from build123d import *

# Parameters (mm, degrees)
SKETCH038_W        = 140
SKETCH038_H        = 93.9
PAD004_DEPTH       = 3
SKETCH039_W        = 12.5
SKETCH039_H        = 38.6472
POCKET028_DEPTH    = 3
SKETCH040_W        = 24
SKETCH040_H        = 60
POCKET029_DEPTH    = 1.5
SKETCH041_R        = 1.05
POCKET030_DEPTH    = 3.001
SKETCH042_R        = 1.9
POCKET031_DEPTH    = 1.4
CHAMFER001_1_ANGLE = 45
CHAMFER001_1_SIZE  = 0.843
CHAMFER001_2_ANGLE = 45
CHAMFER001_2_SIZE  = 0.843
CHAMFER001_3_ANGLE = 45
CHAMFER001_3_SIZE  = 0.843
CHAMFER001_4_ANGLE = 45
CHAMFER001_4_SIZE  = 0.843
FILLET004_R        = 1.5
SKETCH043_R        = 4.85
POCKET032_DEPTH    = 10
FILLET005_R        = 1.8
POCKET033_DEPTH    = 12


with BuildPart() as part:
    # Sketch038 (on XY_Plane154 of Origin468) → Pad004 (new body)
    with BuildSketch(Plane.XY):
        Rectangle(SKETCH038_W, SKETCH038_H)
    extrude(amount=PAD004_DEPTH)

    # Sketch039 (on Face6 of Pad004) → Pocket028 (cut)
    with BuildSketch(Plane.XY.offset(3)):
        Polygon((-61.3, 38.25), (-61.3, -19.25), (-4.3, -19.25), (-4.3, -38.25), (34.2, -38.25), (34.2, 38.25), align=None)
        with Locations((47.48708, -1.86296)):
            Rectangle(SKETCH039_W, SKETCH039_H)
    extrude(amount=-POCKET028_DEPTH, mode=Mode.SUBTRACT)

    # Sketch040 (on Face4 of Pocket028) → Pocket029 (cut)
    with BuildSketch(Plane(origin=(0, 0, 0), x_dir=(1, 0, 0), z_dir=(0, 0, -1))):
        with Locations((48, -11.55)):
            Rectangle(SKETCH040_W, SKETCH040_H)
    extrude(amount=-POCKET029_DEPTH, mode=Mode.SUBTRACT)

    # Sketch041 (on Face5 of Pocket029) → Pocket030 (cut, through all)
    with BuildSketch(Plane.XY.offset(3)):
        with Locations((66.75, 43.7)):
            Circle(SKETCH041_R)
        with Locations((66.75, -43.7)):
            Circle(SKETCH041_R)
        with Locations((-66.75, -43.7)):
            Circle(SKETCH041_R)
        with Locations((-66.75, 43.7)):
            Circle(SKETCH041_R)
    extrude(amount=-POCKET030_DEPTH, mode=Mode.SUBTRACT)

    # Sketch042 (on Face5 of Pocket030) → Pocket031 (cut)
    with BuildSketch(Plane.XY.offset(3)):
        with Locations((-66.75, 43.7)):
            Circle(SKETCH042_R)
        with Locations((66.75, 43.7)):
            Circle(SKETCH042_R)
        with Locations((-66.75, -43.7)):
            Circle(SKETCH042_R)
        with Locations((66.75, -43.7)):
            Circle(SKETCH042_R)
    extrude(amount=-POCKET031_DEPTH, mode=Mode.SUBTRACT)

    # Chamfer001 1
    chamfer001_1_edges = [part.edges().sort_by_distance(p)[0] for p in [
        (-67.8, 43.7, 1.6),
    ]]
    chamfer001_1_side = part.faces().sort_by_distance((-67.8, 43.7, 0.8))[0]
    chamfer(chamfer001_1_edges, length=CHAMFER001_1_SIZE, angle=CHAMFER001_1_ANGLE, reference=chamfer001_1_side)

    # Chamfer001 2
    chamfer001_2_edges = [part.edges().sort_by_distance(p)[0] for p in [
        (65.7, -43.7, 1.6),
    ]]
    chamfer001_2_side = part.faces().sort_by_distance((65.7, -43.7, 0.8))[0]
    chamfer(chamfer001_2_edges, length=CHAMFER001_2_SIZE, angle=CHAMFER001_2_ANGLE, reference=chamfer001_2_side)

    # Chamfer001 3
    chamfer001_3_edges = [part.edges().sort_by_distance(p)[0] for p in [
        (-67.8, -43.7, 1.6),
    ]]
    chamfer001_3_side = part.faces().sort_by_distance((-67.8, -43.7, 0.8))[0]
    chamfer(chamfer001_3_edges, length=CHAMFER001_3_SIZE, angle=CHAMFER001_3_ANGLE, reference=chamfer001_3_side)

    # Chamfer001 4
    chamfer001_4_edges = [part.edges().sort_by_distance(p)[0] for p in [
        (65.7, 43.7, 1.6),
    ]]
    chamfer001_4_side = part.faces().sort_by_distance((65.7, 43.7, 0.8))[0]
    chamfer(chamfer001_4_edges, length=CHAMFER001_4_SIZE, angle=CHAMFER001_4_ANGLE, reference=chamfer001_4_side)

    # Fillet004
    fillet004_edges = [part.edges().sort_by_distance(p)[0] for p in [
        (-4.3, -38.25, 1.5),
        (34.2, -38.25, 1.5),
        (34.2, 38.25, 1.5),
        (-61.3, 38.25, 1.5),
        (-61.3, -19.25, 1.5),
        (-4.3, -19.25, 1.5),
    ]]
    fillet(fillet004_edges, radius=FILLET004_R)

    # Sketch043 (on Face16 of Fillet004) → Pocket032 (cut)
    with BuildSketch(Plane.YZ.offset(70)):
        with Locations((-33.64, -3.85)):
            Circle(SKETCH043_R)
    extrude(amount=-POCKET032_DEPTH, mode=Mode.SUBTRACT)

    # Fillet005
    fillet005_edges = [part.edges().sort_by_distance(p)[0] for p in [
        (70, 0, 3),
        (0, 46.95, 3),
        (70, 46.95, 1.5),
        (-70, 46.95, 1.5),
        (-70, 0, 3),
    ]]
    fillet(fillet005_edges, radius=FILLET005_R)

    # Sketch044 (on Face5 of Fillet005) → Pocket033 (cut)
    with BuildSketch(Plane(origin=(0, 46.95, 0), x_dir=(-1, 0, 0), z_dir=(0, 1, 0))):
        with BuildLine():
            Line((-40.5, -3.1), (-40.5, -0.1))
            ThreePointArc((-40.5, -0.1), (-41.232233, 1.667767), (-43, 2.4))
            Line((-43, 2.4), (-52, 2.4))
            ThreePointArc((-52, 2.4), (-53.767767, 1.667767), (-54.5, -0.1))
            Line((-54.5, -0.1), (-54.5, -3.1))
            ThreePointArc((-54.5, -3.1), (-53.767767, -4.867767), (-52, -5.6))
            Line((-52, -5.6), (-43, -5.6))
            ThreePointArc((-43, -5.6), (-41.232233, -4.867767), (-40.5, -3.1))
        make_face()
    extrude(amount=-POCKET033_DEPTH, mode=Mode.SUBTRACT)


with BuildPart() as part_1:
    # Body003 placement: moved
    add(part.part.moved(Location((-100, 0, 10.5))))


solid = part_1.part
The listing builds one solid part. Answer for the finished solid, in the listing's coordinates (mm). A direction names the side the tool comes from. Round coordinates to 2 decimals unless told otherwise and drop trailing zeros. Write each loop counter-clockwise with the first axis right and the second up, starting at its lowest first coordinate (ties: lowest second). Pieces come first, ordered by that corner, then holes. Notation, with made-up numbers: (83.25, 54.5) - (124.25, 54.5) arc R12 cw to (124.25, 76.5) - close; hole circle Ø7 at (-4, 87.5). An arc over 180 degrees is marked (long way). Use a Markdown table: item, result. Add a question column.
1. For a pull along X with two mould halves and no side action, classify faces 1 (the face through (-161.3, 10, 12)), 2 (the face through (-101, -46.95, 12)) as +X half, -X half, draft (parallel to the pull), parting line (faces both ways), or undercut.
2. The part is cut by section C-C (y = 19). Write down the section's boundary in (x, z), and give its area (3 significant figures).
3. The part is cut by section A-A (y = -16). Write down the section's boundary in (x, z).
4. Flat-ended cylindrical pins translate along their axes: P1, Ø1.9, axis at x = -33.5, y = -43, coming from the +Z side; P2, Ø2.5, axis at x = -33.25, y = 43.7, coming from the +Z side. Find the tip coordinate at first contact, or state that the pin passes through.
5. The part is cut by section D-D (x = -116). Write down the section's boundary in (y, z), and give its area (3 significant figures).
6. Consider line 1 (X direction, y = 7, z = 11.85); line 2 (Y direction, x = -87, z = 10.75); line 3 (Y direction, x = -33.25, z = 12.7). Determine where each line is inside the solid, lowest interval first.
7. The part is cut by section B-B (x = -80.5). Write down the section's boundary in (y, z).
8. A tool of negligible diameter and unlimited length cuts with its end or side. For faces 3 (the face through (-53, 41, 12.9)), 4 (the face through (-117, -20, 10.5)), 5 (the face through (-52, 18, 12)), 6 (the face through (-168.65, 43.78, 12.81)), 7 (the face through (-113, 38.25, 12)), from which of +Z, -Z, +X, -X, +Y, -Y can it reach the whole face along a straight path? Write none if from no direction.
Reported:
| question | item | result |
|---|---|---|
| 1 | face 1 | undercut |
| 1 | face 2 | draft |
| 2 | outline | (-170, 10.5) - (-161.3, 10.5) - (-161.3, 13.5) - (-168.2, 13.5) arc R1.8 ccw to (-170, 11.7) - close; (-65.8, 10.5) - (-64, 10.5) - (-64, 12) - (-40, 12) - (-40, 10.5) - (-30, 10.5) - (-30, 11.7) arc R1.8 ccw to (-31.8, 13.5) - (-65.8, 13.5) - close |
| 2 | area | 96.1 mm^2 |
| 3 | outline | (-170, 10.5) - (-161.3, 10.5) - (-161.3, 13.5) - (-168.2, 13.5) arc R1.8 ccw to (-170, 11.7) - close; (-65.8, 10.5) - (-64, 10.5) - (-64, 12) - (-58.76, 12) - (-58.76, 13.5) - (-65.8, 13.5) - close; (-46.26, 12) - (-40, 12) - (-40, 10.5) - (-30, 10.5) - (-30, 11.7) arc R1.8 ccw to (-31.8, 13.5) - (-46.26, 13.5) - close |
| 4 | P1 | z = 11.9 |
| 4 | P2 | z = 11.46 |
| 5 | outline | (-46.95, 10.5) - (-19.25, 10.5) - (-19.25, 13.5) - (-46.95, 13.5) - close; (38.25, 10.5) - (46.95, 10.5) - (46.95, 11.7) arc R1.8 ccw to (45.15, 13.5) - (38.25, 13.5) - close |
| 5 | area | 109 mm^2 |
| 6 | line 1 | -169.99 to -161.3, -65.8 to -64, -40 to -30.01 |
| 6 | line 2 | -46.95 to -38.25, 38.25 to 46.95 |
| 6 | line 3 | -46.95 to -45.6, -41.8 to 41.8, 45.6 to 46.68 |
| 7 | outline | (-46.95, 10.5) - (-38.25, 10.5) - (-38.25, 13.5) - (-46.95, 13.5) - close; (38.25, 10.5) - (46.95, 10.5) - (46.95, 11.7) arc R1.8 ccw to (45.15, 13.5) - (38.25, 13.5) - close |
| 8 | face 3 | -Z, +Y |
| 8 | face 4 | -Z, +X, -X, +Y, -Y |
| 8 | face 5 | -Z |
| 8 | face 6 | +Z |
| 8 | face 7 | +Z, -Z |
